Answer from the drawing. Dimensions are ordinates in mm from the lowest x, y and z of the part. A direction names the side the tool comes from. Round coordinates to 2 decimals unless told otherwise and drop trailing zeros. Order: outer loops, then holes, each group sorted by start corner. A loop starts at its lowest first (then second) coordinate and runs counter-clockwise, first axis right, second up. Notation, with made-up numbers: (28, 19.5) -> (45, 19.5) arc R20 ccw to (45, 37.5) -> close; hole circle Ø9 at (67, -30.5). An arc over 180 degrees is marked (long way). Use a Markdown table: item, result. Add a question column.
Item 1: A cutting plane is placed at D-D, the plane y = 17.5. Determine the outline of the cut face in (x, z).
Item 2: A tool of negligible diameter and unlimited length cuts with its end or side. For the marked faces 1, 2 and 3, from which of +Z, -Z, +X, -X, +Y, -Y can it reach the whole face along a straight path? Write none if from no direction.
Item 3: A cutting plane is placed at C-C, the plane z = 56. Determine the outline of the cut face in (x, y), plus the area to 3 significant figures.
Item 4: Flat-ended cylindrical pins translate along their axes: P1, Ø8, axis at x = 25.5, z = 75.5, coming from the -Y side; P2, Ø8, axis at y = 42.5, z = 39, coming from the -X side; P3, Ø1, axis at x = 38, z = 82, coming from the +Y side. Find the tip coordinate at first contact, or state that the pin passes through.
Item 5: Find the intervals of material crossed by L1, parallel to Z at x = 66, y = 48.5; L2, parallel to Z at x = 63, y = 64; L3, parallel to X at y = 55.5, z = 102, in increasing order. Write a range as [from, to].
Item 6: A cutting plane is placed at A-A, the plane x = 38.05. Determine the outline of the cut face in (y, z), plus the area to 3 significant figures.
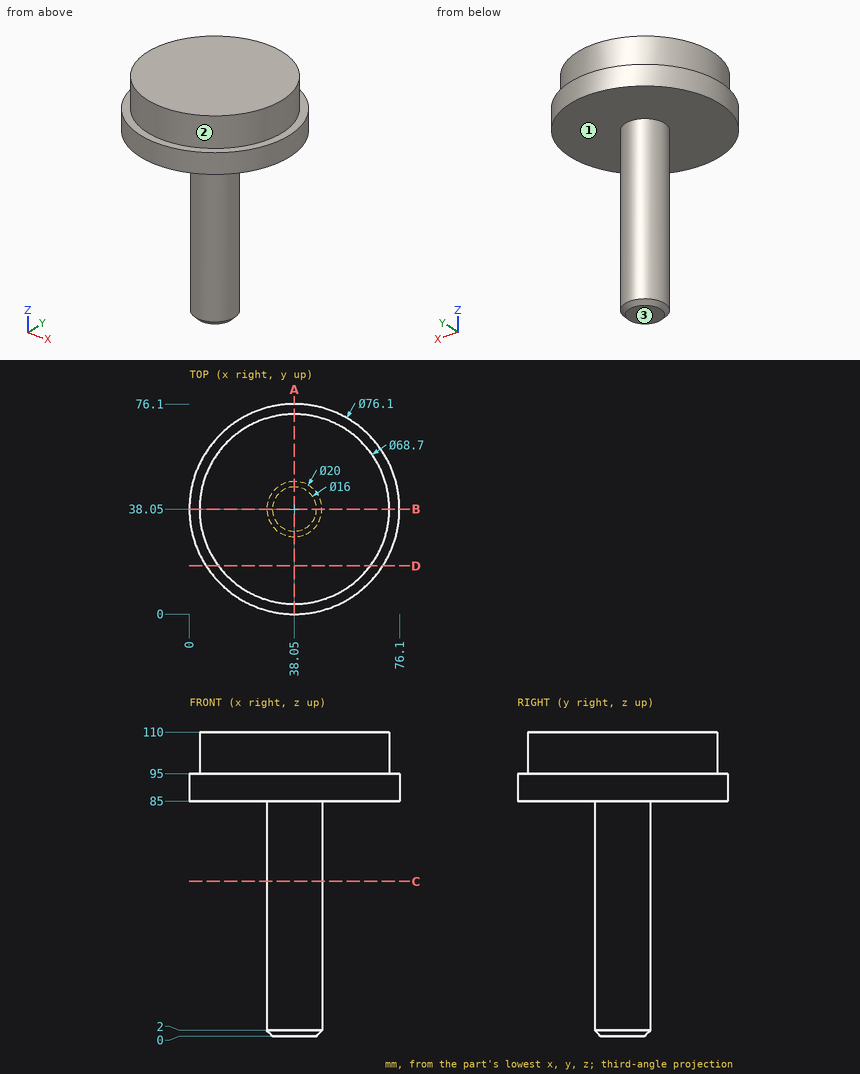
Reported:
| question | item | result |
|---|---|---|
| 1 | outline | (6.03, 85) -> (70.07, 85) -> (70.07, 95) -> (65.57, 95) -> (65.57, 110) -> (10.53, 110) -> (10.53, 95) -> (6.03, 95) -> close |
| 2 | face 1 | -Z |
| 2 | face 2 | +Z |
| 2 | face 3 | -Z, +X, -X, +Y, -Y |
| 3 | outline | circle Ø20 at (38.05, 38.05) |
| 3 | area | 314 mm² |
| 4 | P1 | y = 32.86 |
| 4 | P2 | x = 28.06 |
| 4 | P3 | y = 48.05 |
| 5 | L1 | [85, 110] |
| 5 | L2 | [85, 95] |
| 5 | L3 | [8.46, 67.64] |
| 6 | outline | (0, 85) -> (28.05, 85) -> (28.05, 2) -> (30.05, 0) -> (46.05, 0) -> (48.05, 2) -> (48.05, 85) -> (76.1, 85) -> (76.1, 95) -> (72.4, 95) -> (72.4, 110) -> (3.7, 110) -> (3.7, 95) -> (0, 95) -> close |
| 6 | area | 3,490 mm² |
